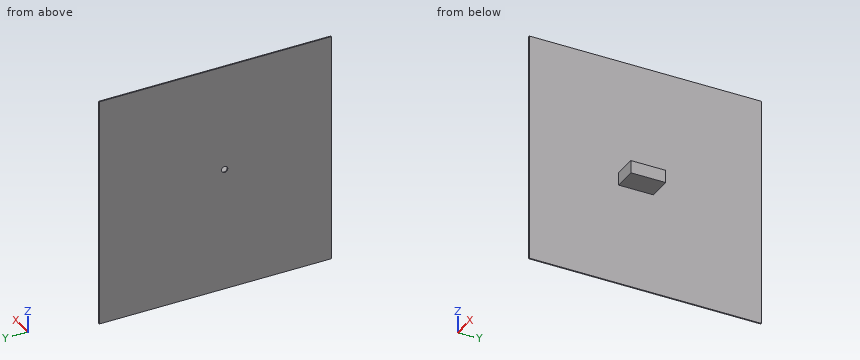
```python
from build123d import *

# Parameters (mm, degrees)
F0_W     = 200
F0_H     = 200
F1_DEPTH = 1
F2_W     = 30
F2_H     = 11
F3_DEPTH = 20
F4_R     = 2.75
F5_DEPTH = 25


with BuildPart() as f1:
    # F0 (on Right) → F1 (new body)
    with BuildSketch(Plane.YZ):
        with Locations((8.036284, 6.124369)):
            Rectangle(F0_W, F0_H)
    extrude(amount=F1_DEPTH)

    # F2 (on face) → F3 (join)
    with BuildSketch(Plane.YZ.offset(1)):
        Rectangle(F2_W, F2_H)
    extrude(amount=F3_DEPTH)

    # F4 (on face) → F5 (cut)
    with BuildSketch(Plane.YZ.offset(1)):
        with Locations((0, 13.5)):
            Circle(F4_R)
    extrude(amount=-F5_DEPTH, mode=Mode.SUBTRACT)


solid = f1.part
```
Build history of the part. All positions in model axes, mm. Round coordinates to 2 decimals unless told otherwise and drop trailing zeros. Loops run counter-clockwise (first coordinate to the right, second up) from the corner with the lowest first, then second, coordinate; pieces in that order, holes last. Notation, with made-up numbers: M -24.5,89 L -14.5,89 A11 cw -14.5,106 Z; hole C 85,84 d7. An arc over 180 degrees is marked long. Answer as CSV lines item,"result".
1. Cut at B-B on z = 13.5. Write the cut outline in (x, y), then the cut area to 4 significant figures.
Resolved:
outline,"M 0,-91.96 L 1,-91.96 L 1,-2.75 L 0,-2.75 Z; M 0,2.75 L 1,2.75 L 1,108.04 L 0,108.04 Z"
area,"194.5 mm²"
2. Wall check: probe 1 along Z at (x, y) = (0.75, 0); probe 2 along X at (y, z) = (29, 35.5); probe 3 along Y at (x, z) = (6, 0). Give the ranges that are in metal, low to high. Write a range as [from, to].
Resolved:
probe 1,"z = [-93.88, 10.75], [16.25, 106.12]"
probe 2,"x = [0, 1]"
probe 3,"y = [-15, 15]"
3. Cut at A-A on y = 0. Write the cut outline in (x, z).
Resolved:
outline,"M 0,-93.88 L 1,-93.88 L 1,-5.5 L 21,-5.5 L 21,5.5 L 1,5.5 L 1,10.75 L 0,10.75 Z; M 0,16.25 L 1,16.25 L 1,106.12 L 0,106.12 Z"
4. Cut at D-D on x = 13.5. Write the cut outline in (y, z).
Resolved:
outline,"M -15,-5.5 L 15,-5.5 L 15,5.5 L -15,5.5 Z"
5. Cut at C-C on y = -65.5. Write the cut outline in (x, z), then the cut area to 3 significant figures.
Resolved:
outline,"M 0,-93.88 L 1,-93.88 L 1,106.12 L 0,106.12 Z"
area,"200 mm²"
6. Flat gauge pins, fed straight in: P1, Ø5.5, axis at x = 12, z = 2, coming from the -Y side; P2, Ø6, axis at x = 15, y = 4.5, coming from the +Z side; P3, Ø12, axis at x = 15.5, z = 0, coming from the +Y side. Where does each tip first touch, or does it go through?
Resolved:
P1,"stops at y = -15"
P2,"stops at z = 5.5"
P3,"stops at y = 15"
